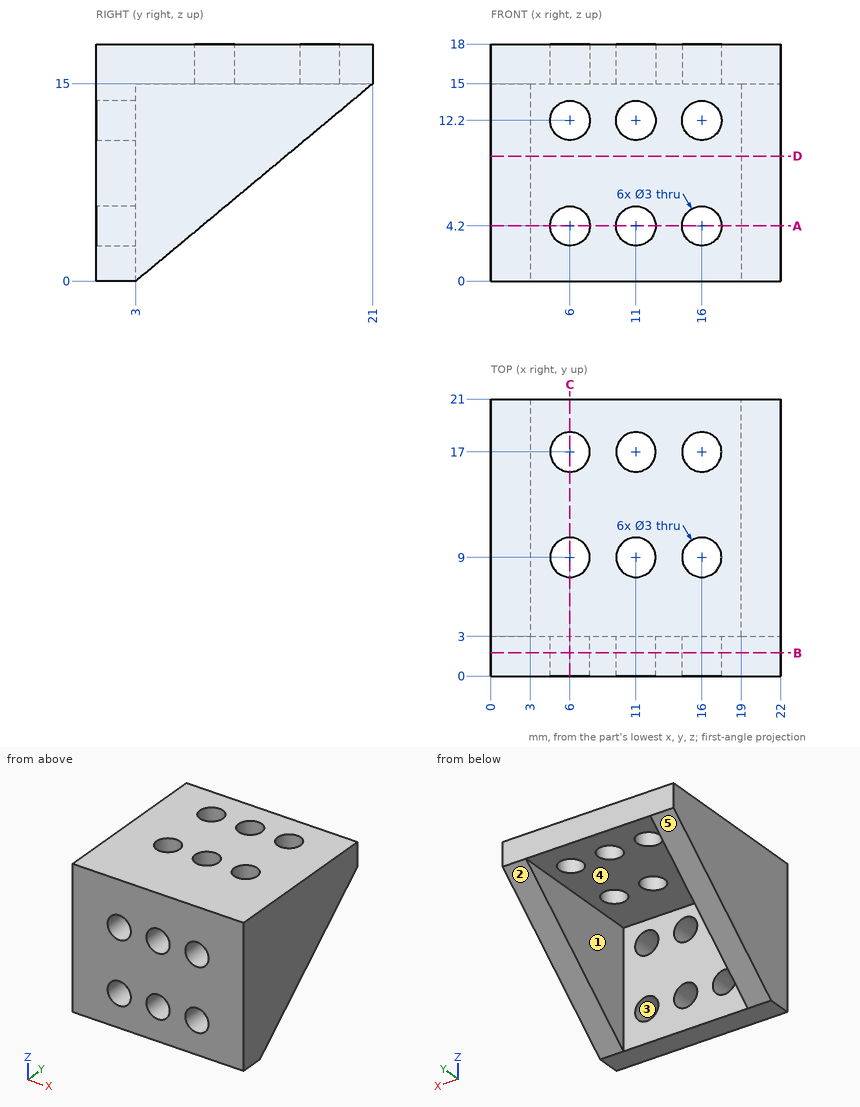
Study the drawing (mm; zero at the part's minimum x, y, z) and answer. A direction names the side the tool comes from. Give positions to 0.01 mm unless a question says otherwise; leave off trailing zeros. Write each loop counter-clockwise with the first axis right and the second up, starting at its lowest first coordinate (ties: lowest second). Pieces come first, ordered by that corner, then holes. Notation, with made-up numbers: (65, 52) - (123, 52) arc R31 ccw to (123, 83) - close; hole circle Ø8 at (-37, -30). An arc over 180 degrees is marked (long way). Write item = value, one per line. Start each with the question number.
Item 1: A tool of negligible diameter and unlimited length cuts with its end or side. For the marked faces 4 and 5, from which of +Z, -Z, +X, -X, +Y, -Y can it reach the whole face along a straight path? Write none if from no direction.
Item 2: The mould has two halves that part along Z. Classify the marked faces 1, 2 and 3: +Z half, -Z half, draft (parallel to the pull), parting line (faces both ways), or undercut.
Item 3: Find the intervals of material crossed by probe 1 along X at (y, z) = (0.95, 4.2); probe 2 along X at (y, z) = (9.5, 9.5); probe 3 along Y at (x, z) = (11.75, 1.5), in increasing order. Write a range as [from, to].
Item 4: Each of these flat-tipped pins is pushed along its axis until it touches: P1, Ø1.8, axis at x = 6, z = 12.2, coming from the +Y side; P2, Ø8, axis at x = 8, y = 16, coming from the -Z side; P3, Ø5, axis at x = 11, z = 4.2, coming from the +Y side. Where does it stop, or does it pass through?
Item 5: Find section B-B (y = 1.75). Give the vertices of the cut face in (x, z), then the cut area to 3 significant figures.
Item 6: Find section A-A (z = 4.2). Give the vertices of the cut face in (x, y).
Item 7: Find section C-C (x = 6). Give the vertices of the cut face in (y, z).
Item 8: Find section D-D (z = 9.5). Give the vertices of the cut face in (x, y), then the cut area to 3 significant figures.
Response:
q1.face_4 = -Z, +Y
q1.face_5 = -Z, +X, -X, +Y
q2.face_1 = draft
q2.face_2 = -Z half
q2.face_3 = undercut
q3.probe_1 = [0, 4.5], [7.5, 9.5], [12.5, 14.5], [17.5, 22]
q3.probe_2 = [0, 3], [19, 22]
q3.probe_3 = [0, 3]
q4.P1 = through
q4.P2 = 15
q4.P3 = 3
q5.outline = (0, 0) - (22, 0) - (22, 18) - (0, 18) - close; hole circle Ø3 at (6, 4.2); hole circle Ø3 at (6, 12.2); hole circle Ø3 at (11, 4.2); hole circle Ø3 at (11, 12.2); hole circle Ø3 at (16, 4.2); hole circle Ø3 at (16, 12.2)
q5.area = 354 mm²
q6.outline = (0, 0) - (4.5, 0) - (4.5, 3) - (3, 3) - (3, 8.04) - (0, 8.04) - close; (7.5, 0) - (9.5, 0) - (9.5, 3) - (7.5, 3) - close; (12.5, 0) - (14.5, 0) - (14.5, 3) - (12.5, 3) - close; (17.5, 0) - (22, 0) - (22, 8.04) - (19, 8.04) - (19, 3) - (17.5, 3) - close
q7.outline = (0, 0) - (3, 0) - (3, 2.7) - (0, 2.7) - close; (0, 5.7) - (3, 5.7) - (3, 10.7) - (0, 10.7) - close; (0, 13.7) - (3, 13.7) - (3, 15) - (7.5, 15) - (7.5, 18) - (0, 18) - close; (10.5, 15) - (15.5, 15) - (15.5, 18) - (10.5, 18) - close; (18.5, 15) - (21, 15) - (21, 18) - (18.5, 18) - close
q8.outline = (0, 0) - (22, 0) - (22, 14.4) - (19, 14.4) - (19, 3) - (3, 3) - (3, 14.4) - (0, 14.4) - close
q8.area = 134 mm²
